from build123d import *

# Parameters (mm, degrees)
RESSALTO_EXTRUS_O3_DEPTH = 10.5


with BuildPart() as part:
    # Esboço2 → Ressalto-extrusão3 (new body)
    with BuildSketch(Plane.XZ.offset(-2101.521299532)):
        with BuildLine():
            Line((1583.190356412, 82.728727741), (1546.151606107, 82.728727741))
            ThreePointArc((1546.151606107, 82.728727741), (1545.285228646, 82.531334214), (1544.589868488, 81.978117836))
            Line((1544.589868488, 81.978117836), (1533.628618793, 68.276555718))
            ThreePointArc((1533.628618793, 68.276555718), (1533.303099773, 67.689179505), (1533.190356412, 67.027165622))
            Line((1533.190356412, 67.027165622), (1533.190356412, 52.082793664))
            ThreePointArc((1533.190356412, 52.082793664), (1533.534221951, 50.961536045), (1534.447575059, 50.225840282))
            Line((1534.447575059, 50.225840282), (1552.832739866, 42.871774359))
            ThreePointArc((1552.832739866, 42.871774359), (1553.197306177, 42.764814968), (1553.575521219, 42.728727741))
            Line((1553.575521219, 42.728727741), (1560.361929287, 42.728727741))
            ThreePointArc((1560.361929287, 42.728727741), (1561.127296152, 42.880968676), (1561.776142849, 43.314514179))
            Line((1561.776142849, 43.314514179), (1562.604569974, 44.142941304))
            ThreePointArc((1562.604569974, 44.142941304), (1563.253416672, 44.576486806), (1564.018783537, 44.728727741))
            Line((1564.018783537, 44.728727741), (1583.190356412, 44.728727741))
            Line((1583.190356412, 44.728727741), (1583.190356412, 82.728727741))
        make_face()
        with BuildLine():
            Line((1564.018783537, 45.228727741), (1582.690356412, 45.228727741))
            Line((1582.690356412, 45.228727741), (1582.690356412, 82.228727741))
            Line((1582.690356412, 82.228727741), (1546.151606107, 82.228727741))
            ThreePointArc((1546.151606107, 82.228727741), (1545.501823011, 82.080682596), (1544.980302893, 81.665770313))
            Line((1544.980302893, 81.665770313), (1534.019053198, 67.964208194))
            ThreePointArc((1534.019053198, 67.964208194), (1533.774913933, 67.523676035), (1533.690356412, 67.027165622))
            Line((1533.690356412, 67.027165622), (1533.690356412, 52.082793664))
            ThreePointArc((1533.690356412, 52.082793664), (1533.948255566, 51.24185045), (1534.633270397, 50.690078628))
            Line((1534.633270397, 50.690078628), (1553.018435204, 43.336012705))
            ThreePointArc((1553.018435204, 43.336012705), (1553.291859937, 43.255793161), (1553.575521219, 43.228727741))
            Line((1553.575521219, 43.228727741), (1560.361929287, 43.228727741))
            ThreePointArc((1560.361929287, 43.228727741), (1560.935954436, 43.342908442), (1561.422589459, 43.668067569))
            Line((1561.422589459, 43.668067569), (1562.251016584, 44.496494694))
            ThreePointArc((1562.251016584, 44.496494694), (1563.062074956, 45.038426572), (1564.018783537, 45.228727741))
        make_face(mode=Mode.SUBTRACT)
    extrude(amount=-RESSALTO_EXTRUS_O3_DEPTH)


solid = part.part
Can you work these out from the model? Positions are in its coordinate system, mm. A direction names the side the tool comes from. Coordinates: 2 decimals unless noted, no trailing zeros. Order: outer loops, then holes, each group sorted by start corner. A loop starts at its lowest first (then second) coordinate and runs counter-clockwise, first axis right, second up. Notation, with made-up numbers: (4, 29) - (45, 29) arc R25 cw to (45, 58) - close; hole circle Ø7 at (61.5, 43.5). An arc over 180 degrees is marked (long way). Answer as a JSON object with one key per item and string values. Group by question number.
Q1. Imagine slicing it at A-A (z = 63.5). Please give me the cut outline in (x, y).
Q2. Imagine slicing it at C-C (y = 2103.75). Please give me the cut outline in (x, z), and give its area (4 significant figures).
Q3. I need wall thicknesses on line 1 (Z direction, x = 1569, y = 2106); line 2 (Z direction, x = 1558, y = 2111.25); line 3 (X direction, y = 2102.5, z = 65). Which ranges of each line are inside material? Lowest first, please. Write a range as from..to.
Q4. We'd pull the mould along Z, two halves only. Please class faces 1 (the face through (1545.3, 2106.7, 82.54)), 2 (the face through (1543.697, 2106.698, 47.065)), 3 (the face through (1563.24, 2106.7, 44.57)): +Z half, -Z half, draft (parallel to the pull), parting line (faces both ways), or undercut.
Q5. On a 3-axis mill with a long thin cutter (end or side, diameter ignored), from which of +Z, -Z, +X, -X, +Y, -Y can I reach the whole of each face in a straight line? I mean faces 4 (the face through (1573, 2107, 45.229)), 5 (the face through (1543.51, 2106.7, 46.6)), 6 (the face through (1573, 2107, 44.729)). Say none if no direction works.
Q6. Imagine slicing it at B-B (x = 1574). Please give me the cut outline in (y, z), and give its area (3 significant figures).
Q7. Will these pins go through, and if not, where does the flat tip stop? P1, Ø2, axis at x = 1563, y = 2106, coming from the -Z side; P2, Ø1.5, axis at y = 2104, z = 74.5, coming from the -X side; P3, Ø5, axis at x = 1566.5, y = 2108, coming from the -Z side.
Determined:
{
 "1": {"outline": "(1533.19, 2101.52) - (1533.69, 2101.52) - (1533.69, 2112.02) - (1533.19, 2112.02) - close; (1582.69, 2101.52) - (1583.19, 2101.52) - (1583.19, 2112.02) - (1582.69, 2112.02) - close"},
 "2": {"outline": "(1533.19, 52.08) arc R2 ccw to (1534.45, 50.23) - (1552.83, 42.87) arc R2 ccw to (1553.58, 42.73) - (1560.36, 42.73) arc R2 ccw to (1561.78, 43.31) - (1562.6, 44.14) arc R2 cw to (1564.02, 44.73) - (1583.19, 44.73) - (1583.19, 82.73) - (1546.15, 82.73) arc R2 ccw to (1544.59, 81.98) - (1533.63, 68.28) arc R2 ccw to (1533.19, 67.03) - close; hole (1533.69, 52.08) arc R1.5 ccw to (1534.63, 50.69) - (1553.02, 43.34) arc R1.5 ccw to (1553.58, 43.23) - (1560.36, 43.23) arc R1.5 ccw to (1561.42, 43.67) - (1562.25, 44.5) arc R2.5 cw to (1564.02, 45.23) - (1582.69, 45.23) - (1582.69, 82.23) - (1546.15, 82.23) arc R1.5 ccw to (1544.98, 81.67) - (1534.02, 67.96) arc R1.5 ccw to (1533.69, 67.03) - close", "area": "81.05 mm2"},
 "3": {"line 1": "z = 44.73..45.23, 82.23..82.73", "line 2": "z = 42.73..43.23, 82.23..82.73", "line 3": "x = 1533.19..1533.69, 1582.69..1583.19"},
 "4": {"face 1": "+Z half", "face 2": "undercut", "face 3": "-Z half"},
 "5": {"face 4": "+Y, -Y", "face 5": "-Z, -X, +Y, -Y", "face 6": "-Z, +X, +Y, -Y"},
 "6": {"outline": "(2101.52, 44.73) - (2112.02, 44.73) - (2112.02, 45.23) - (2101.52, 45.23) - close; (2101.52, 82.23) - (2112.02, 82.23) - (2112.02, 82.73) - (2101.52, 82.73) - close", "area": "10.5 mm2"},
 "7": {"P1": "stops at z = 43.54", "P2": "stops at x = 1538.01", "P3": "stops at z = 44.73"}
}
